Source: CAD feature listing. Evaluate the final solid. Frame: model axes, mm. A direction names the side the tool comes from. Give positions to 0.01 mm unless a question says otherwise; leave off trailing zeros. Order: outer loops, then holes, each group sorted by start corner. A loop starts at its lowest first (then second) coordinate and runs counter-clockwise, first axis right, second up. Notation, with made-up numbers: (-31.75, 41.5) - (-24.75, 41.5) arc R14 cw to (-24.75, 66.5) - close; hole circle Ø5 at (33, 9.25). An arc over 180 degrees is marked (long way). Use CSV: the item, a comma, the result in double quotes.
```python
from build123d import *

# Parameters (mm, degrees)
BOSS_EXTRUDE1_DEPTH = 76.2
SKETCH2_W           = 2.54
SKETCH2_H           = 19.05
BOSS_EXTRUDE2_DEPTH = 76.2
SKETCH3_W           = 17.78
SKETCH3_H           = 17.78
SKETCH3_R           = 6.35
BOSS_EXTRUDE3_DEPTH = 6.35
CUT_EXTRUDE1_DEPTH  = 84.75926815
SKETCH5_W           = 44.45
SKETCH5_H           = 30.48
CUT_EXTRUDE2_DEPTH  = 94.314843428
CUT_EXTRUDE3_START  = -76.2
SKETCH6_W           = 2.54
SKETCH6_H           = 12.08
CUT_EXTRUDE3_DEPTH  = 76.2


with BuildPart() as part:
    # Sketch1 → Boss-Extrude1 (new body)
    with BuildSketch(Plane.XY):
        Polygon((-16.27, 6.97), (16.27, 6.97), (16.27, 12.05), (15, 12.05), (15, 19.05), (16.27, 19.05), (16.27, 21.59), (18.034, 21.59), (18.034, 5.08), (21.209, 5.08), (21.209, 0), (23.749, 0), (23.749, 25.4), (-23.749, 25.4), (-23.749, 0), (-21.209, 0), (-21.209, 5.08), (-18.034, 5.08), (-18.034, 21.59), (-16.27, 21.59), (-16.27, 19.05), (-15, 19.05), (-15, 12.05), (-16.27, 12.05), align=None)
    extrude(amount=BOSS_EXTRUDE1_DEPTH)

    # Sketch2 → Boss-Extrude2 (add)
    with BuildSketch(Plane.XY.offset(76.2)):
        with Locations((-22.479, -4.445)):
            Rectangle(SKETCH2_W, SKETCH2_H)
    extrude(amount=-BOSS_EXTRUDE2_DEPTH)

    # Sketch3 → Boss-Extrude3 (add)
    with BuildSketch(Plane.XY.offset(76.2)):
        with Locations((6.35, -1.92)):
            Rectangle(SKETCH3_W, SKETCH3_H)
        with Locations((6.35, -1.92)):
            Circle(SKETCH3_R, mode=Mode.SUBTRACT)
    boss_extrude3 = extrude(amount=-BOSS_EXTRUDE3_DEPTH)

    # Mirror1: Boss-Extrude3 across plane
    add(boss_extrude3.mirror(Plane.XY.offset(38.1)))

    # Sketch4 → Cut-Extrude1 (cut, through all)
    with BuildSketch(Plane.XY.offset(76.2)):
        Polygon((-6.35, 25.4), (-10.016174209, 19.05), (10.016174209, 19.05), (6.35, 25.4), align=None)
    extrude(amount=-CUT_EXTRUDE1_DEPTH, mode=Mode.SUBTRACT)

    # Sketch5 → Cut-Extrude2 (cut, through all)
    with BuildSketch(Plane(origin=(23.749, 0, 0), x_dir=(0, 0, -1), z_dir=(1, 0, 0))):
        with Locations((-38.1, 1.27)):
            Rectangle(SKETCH5_W, SKETCH5_H)
    extrude(amount=-CUT_EXTRUDE2_DEPTH, mode=Mode.SUBTRACT)

    # Sketch6 → Cut-Extrude3 (cut)
    with BuildSketch(Plane.XY.offset(76.2).offset(CUT_EXTRUDE3_START)):
        with Locations((-15, 13.01)):
            Rectangle(SKETCH6_W, SKETCH6_H)
    extrude(amount=CUT_EXTRUDE3_DEPTH, mode=Mode.SUBTRACT)


solid = part.part
```
Item 1: Section C-C on x = -12. Return the cut outline in (y, z) (3 decimals).
Filled in:
outline,"(6.97, 0) - (25.4, 0) - (25.4, 76.2) - (6.97, 76.2) - (6.97, 60.325) - (16.51, 60.325) - (16.51, 15.875) - (6.97, 15.875) - close"
Item 2: Section A-A on y = -1.92. Return the cut outline in (x, z) (3 decimals), then the cut area to 3 significant figures.
Filled in:
outline,"(-23.749, 0) - (-21.209, 0) - (-21.209, 15.875) - (-23.749, 15.875) - close; (-23.749, 60.325) - (-21.209, 60.325) - (-21.209, 76.2) - (-23.749, 76.2) - close; (-2.54, 0) - (0, 0) - (0, 6.35) - (-2.54, 6.35) - close; (-2.54, 69.85) - (0, 69.85) - (0, 76.2) - (-2.54, 76.2) - close; (12.7, 0) - (15.24, 0) - (15.24, 6.35) - (12.7, 6.35) - close; (12.7, 69.85) - (15.24, 69.85) - (15.24, 76.2) - (12.7, 76.2) - close"
area,"145 mm2"
Item 3: Section B-B on z = 67. Return the cut outline in (x, y).
Filled in:
outline,"(-23.75, -13.97) - (-21.21, -13.97) - (-21.21, 5.08) - (-18.03, 5.08) - (-18.03, 21.59) - (-16.27, 21.59) - (-16.27, 19.05) - (-13.73, 19.05) - (-13.73, 6.97) - (16.27, 6.97) - (16.27, 12.05) - (15, 12.05) - (15, 19.05) - (16.27, 19.05) - (16.27, 21.59) - (18.03, 21.59) - (18.03, 5.08) - (21.21, 5.08) - (21.21, 0) - (23.75, 0) - (23.75, 25.4) - (6.35, 25.4) - (10.02, 19.05) - (-10.02, 19.05) - (-6.35, 25.4) - (-23.75, 25.4) - close"
Item 4: First-contact query: pin 1 (1.6 mm diameter, centred on x = -19.5, z = 8.5, fed in from -Y); pin 2 (1.7 mm diameter, centred on x = 20, z = 45, fed in from -Y); pin 3 (1.9 mm diameter, centred on y = -1, z = 2.5, fed in from +X). Flat tips, straight axial feed; report the tip coordinate or a pass-through.
Filled in:
pin 1,"stops at y = 5.08"
pin 2,"stops at y = 16.51"
pin 3,"stops at x = 15.24"
Item 5: Set-up query: faces 4 (the flat face through (0, 0, 69.85)), 5 (the flat face through (-20, 5.08, 8)), 6 (the flat face through (21, 10, 15.875)). Return all of +Z, -Z, +X, -X, +Y, -Y with unobstructed straight access to the full face (end or side cutting, diameter ignored); none if empty.
Filled in:
face 4,"-Y"
face 5,"+Z, -Z, -Y"
face 6,"+X, -X, -Y"
Item 6: Material intervals for line 1 (Y direction, x = 6, z = 1); line 2 (Z direction, x = 10, y = 4); line 3 (X direction, y = -1, z = 2), sorted ascending. Write a range as from..to.
Filled in:
line 1,"y = -10.81..-8.26, 4.42..19.05"
line 2,"z = 0..6.35, 69.85..76.2"
line 3,"x = -23.75..-21.21, -2.54..0.07, 12.63..15.24"
Item 7: Section D-D on x = 7.5. Return the cut outline in (y, z) (3 decimals).
Filled in:
outline,"(-10.81, 0) - (-8.165, 0) - (-8.165, 6.35) - (-10.81, 6.35) - close; (-10.81, 69.85) - (-8.165, 69.85) - (-8.165, 76.2) - (-10.81, 76.2) - close; (4.325, 0) - (19.05, 0) - (19.05, 76.2) - (4.325, 76.2) - (4.325, 69.85) - (6.97, 69.85) - (6.97, 60.325) - (16.51, 60.325) - (16.51, 15.875) - (6.97, 15.875) - (6.97, 6.35) - (4.325, 6.35) - close; (23.408, 0) - (25.4, 0) - (25.4, 76.2) - (23.408, 76.2) - close"
Item 8: Mould query, pull axis X, two halves, no side actions, for faces 1 (the flat face through (0, 19.05, 39)), 2 (the flat face through (1, 12, 60.325)), 3 (the flat face through (-23.749, 19, 39)). Classes: released by +X, released by -X, zero draft, split by the parting line, or undercut.
Filled in:
face 1,"undercut"
face 2,"zero draft"
face 3,"released by -X"
